Geometry: final body of the model. Coordinates: model frame, mm. Give positions to 0.01 mm unless a question says otherwise; leave off trailing zeros. Loops run counter-clockwise (first coordinate to the right, second up) from the corner with the lowest first, then second, coordinate; pieces in that order, holes last.
Autodesk Inventor part; units mm, degrees
ref_plane "YZ Plane" through (0, 0, 0) normal (1, 0, 0) x (0, 1, 0)
ref_plane "XZ Plane" through (0, 0, 0) normal (0, 1, 0) x (-1, 0, 0)
ref_plane "XY Plane" through (0, 0, 0) normal (0, 0, 1) x (1, 0, 0)
sketch "Sketch6" plane through (0, 0, 0) normal (0, 1, 0) x (-1, 0, 0)
  line L0 (0, 0) -> (-60.1073, 0)
  line L1 (-60.1073, 0) -> (-60.1073, 2100)
  line L2 (-60.1073, 2100) -> (0, 2100)
  line L3 (0, 2100) -> (0, 0)
  dimension "d26" = 60.1073
  dimension "d27" = 2100
extrude "Plate4" add sketch "Sketch6" along normal blind 3
sketch "Sketch9" plane through (0, 3, 0) normal (0, 1, 0) x (1, 0, 0)
  line L0 (0, -2100) -> (0, 0)
  line L1 (60.1073, -2100) -> (0, -2100)
  line L2 (60.1073, 0) -> (60.1073, -2100)
  line L3 (0, 0) -> (60.1073, 0)
  line L4 (25, -210) -> (10, -210) construction
  line L5 (10, -210) -> (10, -10) construction
  line L6 (10, -10) -> (25, -10) construction
  line L7 (25, -10) -> (25, -210) construction
  dimension "d44" = 200
  dimension "d45" = 15
  dimension "d46" = 10
  dimension "d47" = 10
mark "Mark1"
sketch "Sketch7" plane through (0, 0, 0) normal (0, -1, 0) x (1, 0, 0)
  line L0 (0, 2100) -> (60.1073, 2100)
  line L1 (0, 0) -> (0, 2100)
  line L2 (60.1073, 0) -> (0, 0)
  line L3 (60.1073, 2100) -> (60.1073, 0)
  line L4 (0, 235.2) -> (31.0536, 235.2)
  line L5 (31.0536, 235.2) -> (31.0536, 232)
  line L6 (31.0536, 232) -> (0, 232)
  line L7 (0, 232) -> (0, 235.2)
  point P0 (0, 232)
  point P1 (0, 200)
  point P2 (46.4173, 200)
  point P3 (0, 232)
  dimension "d29" = 31.0536
  dimension "d30" = 3.2
  dimension "d31" = 232
extrude "Extrusion2" cut sketch "Sketch7" against normal through all contours L4 L5 L6 L1
pattern_linear "Rectangular Pattern1" count 5 spacing 500 along (0, 0, 1) of "Extrusion2"
sketch "Sketch8" plane through (0, 0, 0) normal (0, -1, 0) x (1, 0, 0)
  line L0 (0, 1735.2) -> (0, 2100)
  line L1 (0, 235.2) -> (31.0536, 235.2)
  line L2 (31.0536, 235.2) -> (31.0536, 232)
  line L3 (31.0536, 232) -> (0, 232)
  line L4 (0, 0) -> (0, 232)
  line L5 (60.1073, 0) -> (0, 0)
  line L6 (60.1073, 2100) -> (60.1073, 0)
  line L7 (0, 2100) -> (60.1073, 2100)
  circle A0 centre (0, 620) radius 25
  line L8 (0, 1735.2) -> (31.0536, 1735.2)
  line L9 (31.0536, 1735.2) -> (31.0536, 1732)
  line L10 (31.0536, 1732) -> (0, 1732)
  line L11 (0, 1235.2) -> (0, 1732)
  line L12 (0, 1235.2) -> (31.0536, 1235.2)
  line L13 (31.0536, 1235.2) -> (31.0536, 1232)
  line L14 (31.0536, 1232) -> (0, 1232)
  line L15 (0, 735.2) -> (0, 1232)
  line L16 (0, 735.2) -> (31.0536, 735.2)
  line L17 (31.0536, 735.2) -> (31.0536, 732)
  line L18 (31.0536, 732) -> (0, 732)
  line L19 (0, 235.2) -> (0, 732)
  dimension "d37" = 50
  dimension "d38" = 620
extrude "Extrusion3" cut sketch "Sketch8" against normal through all contours L19 A0 | A0 L19
pattern_linear "Rectangular Pattern2" count 2 spacing 1480 along (0, 0, 1) of "Extrusion3"
chamfer "Corner Chamfer1" distance 6 angle 45 2 edges at (25, 1.5, 2100) (60.1073, 1.5, 2100)
equation "\"d26\" = Stringer4_deep"
equation "\"d28\" = Thickness"
equation "\"BendReliefWidth\" = Thickness"
equation "\"BendReliefDepth\" = 0.5 * Thickness"
equation "\"CornerReliefSize\" = 4 * Thickness"
equation "\"MinimumRemnant\" = 2 * Thickness"
equation "\"TransitionRadius\" = BendRadius"
equation "\"JacobiRadiusSize\" = BendRadius"
equation "\"GapSize\" = Thickness"
properties part number "BSH 0363 stringer board 4" material "09g2s"
Item 1: Section query B-B on z = 620. Return loops of the section in (x, y).
Values follow:
outline: (25, 0) - (60.11, 0) - (60.11, 3) - (25, 3) - close
Item 2: Section query A-A on y = 2.1. Return loops of the section in (x, z), plus the area to 3 significant figures.
Values follow:
outline: (0, 0) - (60.11, 0) - (60.11, 2094) - (54.11, 2100) - (31, 2100) - (24.28, 2094.04) arc R25 cw to (0, 2075) - (0, 1735.2) - (31.05, 1735.2) - (31.05, 1732) - (0, 1732) - (0, 1235.2) - (31.05, 1235.2) - (31.05, 1232) - (0, 1232) - (0, 735.2) - (31.05, 735.2) - (31.05, 732) - (0, 732) - (0, 645) arc R25 cw to (0, 595) - (0, 235.2) - (31.05, 235.2) - (31.05, 232) - (0, 232) - close
area: 124,000 mm2
Item 3: Ray query, probe 1 along Z at (x, y) = (18, 0.75); probe 2 along Z at (x, y) = (7.5, 2.75); probe 3 along Z at (x, y) = (27.5, 0.8). Return the intervals inside material, ascending.
Values follow:
probe 1: z = 0 to 232, 235.2 to 602.65, 637.35 to 732, 735.2 to 1232, 1235.2 to 1732, 1735.2 to 2082.65
probe 2: z = 0 to 232, 235.2 to 596.15, 643.85 to 732, 735.2 to 1232, 1235.2 to 1732, 1735.2 to 2076.15
probe 3: z = 0 to 232, 235.2 to 732, 735.2 to 1232, 1235.2 to 1732, 1735.2 to 2096.9
Item 4: Pin query (flat end, axial travel): pin 1 (0.9 mm diameter, centred on x = 14, y = 1, fed in from +Z); pin 2 (0.9 mm diameter, centred on y = 1.5, z = 233.5, fed in from -X); pin 3 (1.5 mm diameter, centred on x = 12.5, y = 2, fed in from +Z). Return the tip coordinate at first contact, or that it passes through.
Values follow:
pin 1: stops at z = 2079.6
pin 2: stops at x = 31.05
pin 3: stops at z = 2078.8
